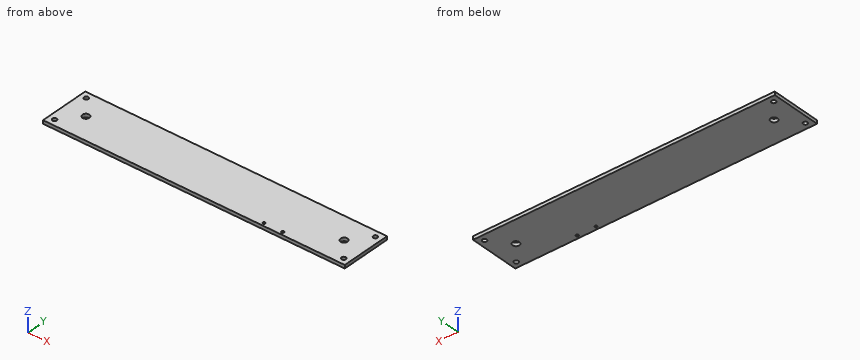
from build123d import *

# Parameters (mm, degrees)
SKETCH1_W           = 360
SKETCH1_H           = 60
SKETCH1_R           = 4.1
SKETCH1_R_2         = 2.55
BOSS_EXTRUDE1_DEPTH = 4
SKETCH3_R           = 1.55
CUT_EXTRUDE2_DEPTH  = 4


with BuildPart() as part:
    # Sketch1 → Boss-Extrude1 (new body)
    with BuildSketch(Plane.XY):
        with Locations((154.041275094, 0)):
            Rectangle(SKETCH1_W, SKETCH1_H)
        Circle(SKETCH1_R, mode=Mode.SUBTRACT)
        with Locations((308, 0)):
            Circle(SKETCH1_R, mode=Mode.SUBTRACT)
        with Locations((-18.451377883, 22.492652976)):
            Circle(SKETCH1_R_2, mode=Mode.SUBTRACT)
        with Locations((-18.451377883, -22.492652976)):
            Circle(SKETCH1_R_2, mode=Mode.SUBTRACT)
        with Locations((326.53392807, 22.492652976)):
            Circle(SKETCH1_R_2, mode=Mode.SUBTRACT)
        with Locations((326.53392807, -22.492652976)):
            Circle(SKETCH1_R_2, mode=Mode.SUBTRACT)
    extrude(amount=BOSS_EXTRUDE1_DEPTH)

    # Sketch3 → Cut-Extrude2 (cut)
    with BuildSketch(Plane.XY.offset(4)):
        with Locations((256.65, -26)):
            Circle(SKETCH3_R)
        with Locations((234.35, -26)):
            Circle(SKETCH3_R)
    extrude(amount=-CUT_EXTRUDE2_DEPTH, mode=Mode.SUBTRACT)


solid = part.part
Verification items for the finished model (mm, model axes). Give positions to 0.01 mm unless a question says otherwise; leave off trailing zeros. Order: outer loops, then holes, each group sorted by start corner. A loop starts at its lowest first (then second) coordinate and runs counter-clockwise, first axis right, second up. Notation, with made-up numbers: M -30.75,-29 L 16.25,-29 A19 ccw 16.25,-25 Z; hole C 59,-18 d9. An arc over 180 degrees is marked long. Answer as a JSON object with one key per item and string values. Group by question number.
1) Depth check by flat-ended pin: pin 1 Ø3 at (x, y) = (326.53, 22.49) entering from -Z. Enter the tip coordinate at first touch or a pass-through.
2) Cross-section at A-A (x = 0). Enter the section's corners in (y, z), then the cut area to 3 significant figures.
3) Scan lines: line 1 along Y through (x, z) = (308, 1.95); line 2 along X through (y, z) = (-21.5, 2.15); line 3 along X through (y, z) = (2, 2.3). Record each from-to range of solid material in increasing order. Write a range as [from, to].
Result sheet:
{
 "1": {"pin 1": "passes through"},
 "2": {"outline": "M -30,0 L -4.1,0 L -4.1,4 L -30,4 Z; M 4.1,0 L 30,0 L 30,4 L 4.1,4 Z", "area": "207 mm2"},
 "3": {"line 1": "y = [-30, -4.1], [4.1, 30]", "line 2": "x = [-25.96, -20.8], [-16.1, 324.19], [328.88, 334.04]", "line 3": "x = [-25.96, -3.58], [3.58, 304.42], [311.58, 334.04]"}
}
